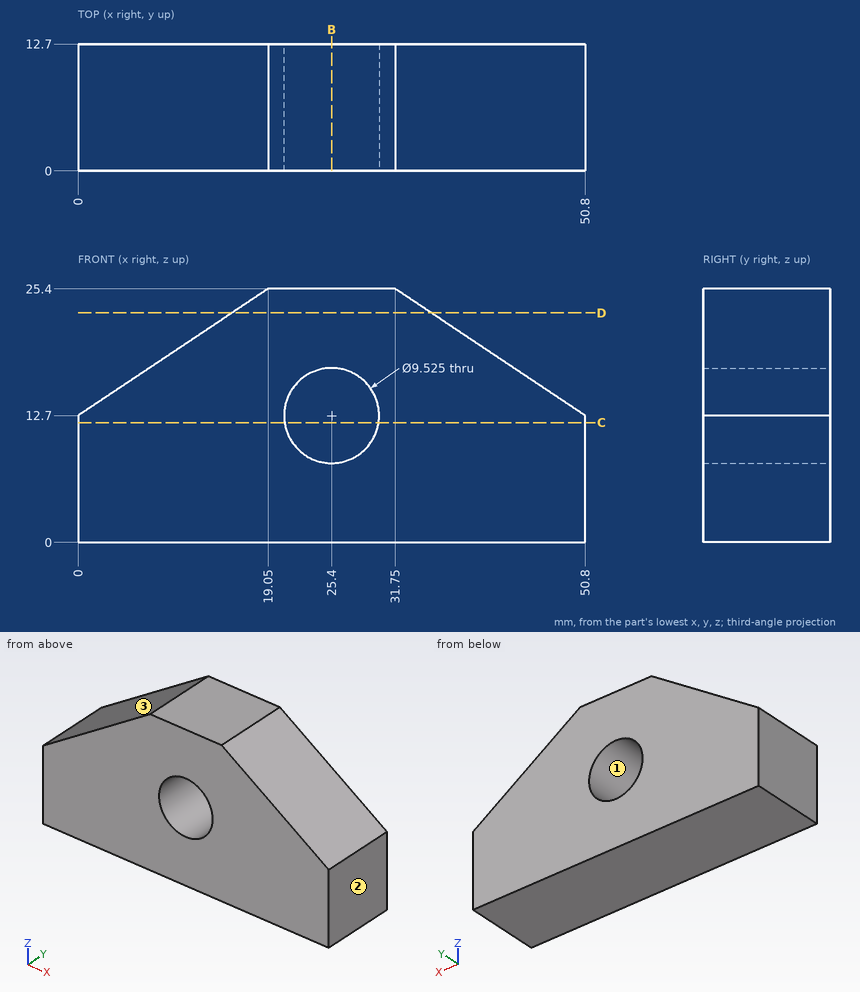
For this review, use the dimensioned drawing (mm, ordinates from the lowest corner) and the shaded views. Round coordinates to 2 decimals unless told otherwise and drop trailing zeros. Order: outer loops, then holes, each group sorted by start corner. A loop starts at its lowest first (then second) coordinate and runs counter-clockwise, first axis right, second up. Notation, with made-up numbers: M 27.25,-40 L 44.25,-40 A11 ccw 44.25,-35 Z; hole C 77.25,42.5 d11. An arc over 180 degrees is marked long. Write each question's results on one line, items separated by ' | '. Start each with the question number.
1. Clearance check with a flat-ended pin moving along its axis: pin 1 Ø1 at (x, y) = (42, 1.5) entering from +Z. State where the tip first meets the part, or that it passes through.
2. To check wall thickness, follow L1, parallel to Z at x = 25.4, y = 7.75; L2, parallel to Z at x = 29, y = 2; L3, parallel to X at y = 12.25, z = 10.25. State the ranges of each line that lie inside material, in increasing order. Write a range as [from, to].
3. Add section B-B (x = 25.4). State the section outline as (y, z) points.
4. Add section D-D (z = 23). State the section outline as (x, y) points, then the cut area to 3 significant figures.
5. Add section C-C (z = 12). State the section outline as (x, y) points.
6. Draft analysis for pull direction X (two halves, no side actions). For the marked faces 1, 2 and 3, state which applies: pulls with the +X half, pulls with the -X half, needs draft (parallel to the pull), parting line crosses it, or undercut.
Output values:
1) pin 1: z = 18.9
2) L1: [0, 7.94], [17.46, 25.4] | L2: [0, 9.58], [15.82, 25.4] | L3: [0, 21.32], [29.48, 50.8]
3) outline: M 0,0 L 12.7,0 L 12.7,7.94 L 0,7.94 Z; M 0,17.46 L 12.7,17.46 L 12.7,25.4 L 0,25.4 Z
4) outline: M 15.45,0 L 35.35,0 L 35.35,12.7 L 15.45,12.7 Z | area: 253 mm^2
5) outline: M 0,0 L 20.69,0 L 20.69,12.7 L 0,12.7 Z; M 30.11,0 L 50.8,0 L 50.8,12.7 L 30.11,12.7 Z
6) face 1: undercut | face 2: pulls with the +X half | face 3: pulls with the -X half
